Input: part model. Units: mm. Frame: model coordinates. Round coordinates to 2 decimals unless told otherwise and drop trailing zeros. Loops run counter-clockwise (first coordinate to the right, second up) from the corner with the lowest first, then second, coordinate; pieces in that order, holes last. Notation, with made-up numbers: (60.5, 0) -> (118.5, 0) arc R32 cw to (118.5, 37) -> close; hole circle Ø3 at (70, 31). An arc over 180 degrees is marked (long way). Answer in a Markdown table with one row per item. Add a question column.
Q1. Section A-A, the plane y = 26. Output: boundary loops of the cut face in (x, z), and give its area (3 significant figures).
Q2. Section C-C, the plane y = 71.5. Output: boundary loops of the cut face in (x, z).
Q3. Section B-B, the plane z = -58. Output: boundary loops of the cut face in (x, y), and give its area (3 significant figures).
Q4. Pin query (flat end, axial travel): pin 1 (3 mm diameter, centred on y = 73.5, z = 38.5, fed in from +X); pin 2 (4 mm diameter, centred on y = 37, z = 22, fed in from -X). Return the tip coordinate at first contact, or that it passes through.
Q5. Ray query, L1, parallel to X at y = 63, z = -51. Return the intervals inside material, ascending. Write a range as from..to.
```python
from build123d import *

# Parameters (mm, degrees)
SKETCH1_W           = 200
SKETCH1_H           = 150
BOSS_EXTRUDE1_DEPTH = 90
SKETCH2_R           = 5.778007253
SKETCH2_R_2         = 6.144226379
SKETCH2_R_3         = 5.765469067
SKETCH2_R_4         = 5.780094306
BOSS_EXTRUDE2_DEPTH = 5
BOSS_EXTRUDE3_START = -205
SKETCH2_2_R         = 5.778007253
SKETCH2_2_R_2       = 6.144226379
SKETCH2_2_R_3       = 5.765469067
SKETCH2_2_R_4       = 5.780094306
BOSS_EXTRUDE3_DEPTH = 5


with BuildPart() as part:
    # Sketch1 → Boss-Extrude1 (new body)
    with BuildSketch(Plane(origin=(0, 0, 0), x_dir=(1, 0, 0), z_dir=(0, 1, 0))):
        Rectangle(SKETCH1_W, SKETCH1_H)
    extrude(amount=BOSS_EXTRUDE1_DEPTH)

    # Sketch2 → Boss-Extrude2 (add)
    with BuildSketch(Plane.ZY.offset(100)):
        with Locations(Location((58.863929125, 11.762847407, 0), (0, 0, 180))):
            Circle(SKETCH2_R)
        with Locations(Location((58.863929125, 28.847365095, 0), (0, 0, 180))):
            Circle(SKETCH2_R_2)
        with Locations(Location((58.863929125, 45.155313797, 0), (0, 0, 180))):
            Circle(SKETCH2_R_3)
        with Locations(Location((58.863929125, 62.084517688, 0), (0, 0, 180))):
            Circle(SKETCH2_R_4)
    extrude(amount=BOSS_EXTRUDE2_DEPTH)

    # Sketch2_2 → Boss-Extrude3 (add)
    with BuildSketch(Plane.ZY.offset(100).offset(BOSS_EXTRUDE3_START)):
        with Locations(Location((58.863929125, 11.762847407, 0), (0, 0, 180))):
            Circle(SKETCH2_2_R)
        with Locations(Location((58.863929125, 28.847365095, 0), (0, 0, 180))):
            Circle(SKETCH2_2_R_2)
        with Locations(Location((58.863929125, 45.155313797, 0), (0, 0, 180))):
            Circle(SKETCH2_2_R_3)
        with Locations(Location((58.863929125, 62.084517688, 0), (0, 0, 180))):
            Circle(SKETCH2_2_R_4)
    extrude(amount=BOSS_EXTRUDE3_DEPTH)


solid = part.part
```
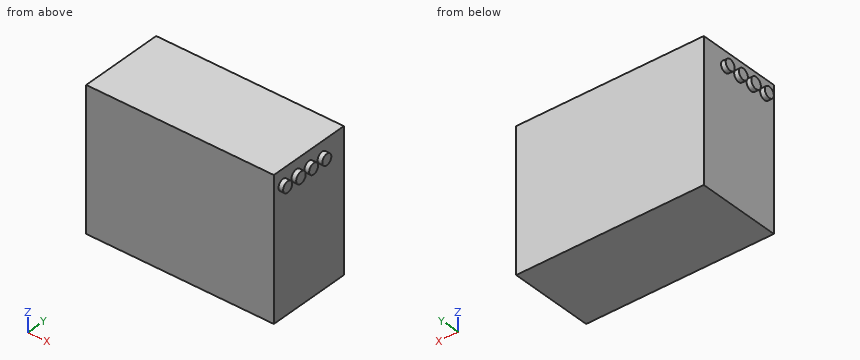
Answer block:
| question | item | result |
|---|---|---|
| 1 | outline | (-105, 53.42) -> (-100, 53.42) -> (-100, -75) -> (100, -75) -> (100, 53.42) -> (105, 53.42) -> (105, 64.31) -> (100, 64.31) -> (100, 75) -> (-100, 75) -> (-100, 64.31) -> (-105, 64.31) -> close |
| 1 | area | 30,100 mm^2 |
| 2 | outline | (-100, -75) -> (100, -75) -> (100, 75) -> (-100, 75) -> close |
| 3 | outline | (-100, 0) -> (100, 0) -> (100, 90) -> (-100, 90) -> close |
| 3 | area | 18,000 mm^2 |
| 4 | pin 1 | x = 100 |
| 4 | pin 2 | x = -100 |
| 5 | L1 | -100..100 |
